```python
from build123d import *

# Parameters (mm, degrees)
SKICA1_W                 = 14.9
SKICA1_H                 = 11.7
P_IDAT_VYSUNUT_M1_DEPTH  = 11.7
ODEBRAT_VYSUNUT_M2_DEPTH = 2.3
ODEBRAT_VYSUNUT_M3_DEPTH = 20
ZAOBLIT2_R               = 0.8
SKICA9_W                 = 8.55
SKICA9_H                 = 3.05
P_IDAT_VYSUNUT_M3_DEPTH  = 5.6
ZAOBLIT3_R               = 4.25
SKICA10_W                = 8.55
SKICA10_H                = 3.05
P_IDAT_VYSUNUT_M4_DEPTH  = 5.6
ZAOBLIT4_R               = 4.25


with BuildPart() as part:
    # Skica1 → Přidat vysunutím1 (new body)
    with BuildSketch(Plane.XY):
        Rectangle(SKICA1_W, SKICA1_H)
    extrude(amount=P_IDAT_VYSUNUT_M1_DEPTH)

    # Skica2 → Odebrat vysunutím2 (cut)
    with BuildSketch(Plane.XY.offset(11.7)):
        with BuildLine():
            Line((-5.65, -5.85), (5.65, -5.85))
            Line((5.65, -5.85), (5.65, 2.7))
            ThreePointArc((5.65, 2.7), (5.254594155, 3.654594155), (4.3, 4.05))
            Line((4.3, 4.05), (-4.3, 4.05))
            ThreePointArc((-4.3, 4.05), (-5.254594155, 3.654594155), (-5.65, 2.7))
            Line((-5.65, 2.7), (-5.65, -5.85))
        make_face()
    extrude(amount=-ODEBRAT_VYSUNUT_M2_DEPTH, mode=Mode.SUBTRACT)

    # Skica5 → Odebrat vysunutím3 (cut)
    with BuildSketch(Plane.XY.offset(9.4)):
        Polygon((-4.3, 4.05), (4.3, 4.05), (5.65, 4.05), (5.65, -5.85), (-5.65, -5.85), (-5.65, 4.05), align=None)
    extrude(amount=-ODEBRAT_VYSUNUT_M3_DEPTH, mode=Mode.SUBTRACT)

    # Zaoblit2
    zaoblit2_edges = [part.edges().sort_by_distance(p)[0] for p in [
        (-7.45, 5.85, 5.85),
        (7.45, 5.85, 5.85),
    ]]
    fillet(zaoblit2_edges, radius=ZAOBLIT2_R)

    # Skica9 → Přidat vysunutím3 (add)
    with BuildSketch(Plane.ZY.offset(7.45)):
        with Locations((4.275, -4.325)):
            Rectangle(SKICA9_W, SKICA9_H)
    extrude(amount=P_IDAT_VYSUNUT_M3_DEPTH)

    # Zaoblit3
    zaoblit3_edges = [part.edges().sort_by_distance(p)[0] for p in [
        (-13.05, -4.325, 0),
        (-13.05, -4.325, 8.55),
    ]]
    fillet(zaoblit3_edges, radius=ZAOBLIT3_R)

    # Skica10 → Přidat vysunutím4 (add)
    with BuildSketch(Plane(origin=(7.45, 0, 0), x_dir=(0, 0, -1), z_dir=(1, 0, 0))):
        with Locations((-4.275, -4.325)):
            Rectangle(SKICA10_W, SKICA10_H)
    extrude(amount=P_IDAT_VYSUNUT_M4_DEPTH)

    # Zaoblit4
    zaoblit4_edges = [part.edges().sort_by_distance(p)[0] for p in [
        (13.05, -4.325, 8.55),
        (13.05, -4.325, 0),
    ]]
    fillet(zaoblit4_edges, radius=ZAOBLIT4_R)


solid = part.part
```
Could you check a few things on this model? Use its own coordinates, in mm. A direction names the side the tool comes from. Round coordinates to 2 decimals unless told otherwise and drop trailing zeros. Write each loop counter-clockwise with the first axis right and the second up, starting at its lowest first coordinate (ties: lowest second). Pieces come first, ordered by that corner, then holes. Notation, with made-up numbers: M -9.5,-24.5 L 19.5,-24.5 A20 cw 19.5,14.5 Z; hole C 42,3 d7. An arc over 180 degrees is marked long. Answer in a Markdown table with one row per item. Add a question column.
Q1. Imagine slicing it at B-B (y = 0.5). Please give me the cut outline in (x, z), then the cut area to 3 significant figures.
Q2. Will these pins go through, and if not, where does the flat tip stop? pin 1 Ø3 at (y, z) = (-3, 7) entering from +X; pin 2 Ø4.5 at (x, z) = (-10.5, 3) entering from +Y; pin 3 Ø4.5 at (x, z) = (9, 3) entering from +Y.
Q3. If I drill on line 1 (X direction, y = 2, z = 11); line 2 (Y direction, x = 12, z = 4.75); line 3 (Y direction, x = -3.5, z = 4), over which ranges is the centre line in solid material (lowest first)? Write a range as from..to.
Q4. Imagine slicing it at A-A (y = -3.25). Please give me the cut outline in (x, z).
Q5. Imagine slicing it at D-D (x = -8). Please give me the cut outline in (y, z).
Q6. On a 3-axis mill with a long thin cutter (end or side, diameter ignored), from which of +Z, -Z, +X, -X, +Y, -Y can I reach the whole of each face in a straight line? I mean faces 1 (the cylindrical face through (5.27, 3.64, 10.57)), 2 (the flat face through (8, -4, 8.55)), 3 (the flat face through (-10, -2.8, 4)), 4 (the flat face through (0, 4.05, 6)), 5 (the flat face through (10, -2.8, 4)). Say none if no direction works.
Q7. If we mould it in two halves opening along X, with no side actions, what happens to faces 6 (the cylindrical face through (11.77, -4.3, 7.34)), 7 (the flat face through (-5.4, 3.8, 9.4)), 8 (the flat face through (0, 5.85, 6))? For each: +X half, -X half, draft (parallel to the pull), parting line (faces both ways), or undercut.
Q8. Imagine slicing it at C-C (z = 2.5). Please give me the cut outline in (x, y).
Values:
| question | item | result |
|---|---|---|
| 1 | outline | M -7.45,0 L -5.65,0 L -5.65,11.7 L -7.45,11.7 Z; M 5.65,0 L 7.45,0 L 7.45,11.7 L 5.65,11.7 Z |
| 1 | area | 42.1 mm^2 |
| 2 | pin 1 | x = 12.88 |
| 2 | pin 2 | y = -2.8 |
| 2 | pin 3 | y = 5.84 |
| 3 | line 1 | -7.45..-5.65, 5.65..7.45 |
| 3 | line 2 | -5.85..-2.8 |
| 3 | line 3 | 4.05..5.85 |
| 4 | outline | M -13.05,4.25 A4.25 ccw -8.8,0 L -5.65,0 L -5.65,11.7 L -7.45,11.7 L -7.45,8.55 L -8.8,8.55 A4.25 ccw -13.05,4.3 Z; M 5.65,0 L 8.8,0 A4.25 ccw 13.05,4.25 L 13.05,4.3 A4.25 ccw 8.8,8.55 L 7.45,8.55 L 7.45,11.7 L 5.65,11.7 Z |
| 5 | outline | M -5.85,0 L -2.8,0 L -2.8,8.55 L -5.85,8.55 Z |
| 6 | face 1 | +Z, -Z, -Y |
| 6 | face 2 | +Z, +X, +Y, -Y |
| 6 | face 3 | +Z, -Z, -X, +Y |
| 6 | face 4 | -Z, -Y |
| 6 | face 5 | +Z, -Z, +X, +Y |
| 7 | face 6 | +X half |
| 7 | face 7 | undercut |
| 7 | face 8 | draft |
| 8 | outline | M -12.67,-5.85 L -5.65,-5.85 L -5.65,4.05 L 5.65,4.05 L 5.65,-5.85 L 12.67,-5.85 L 12.67,-2.8 L 7.45,-2.8 L 7.45,5.05 A0.8 ccw 6.65,5.85 L -6.65,5.85 A0.8 ccw -7.45,5.05 L -7.45,-2.8 L -12.67,-2.8 Z |
